Design review of the part built by this model. Coordinates are the model's own, in mm. Face numbers are marked on the shaded views. A direction names the side the tool comes from. Round coordinates to 2 decimals unless told otherwise and drop trailing zeros. Order: outer loops, then holes, each group sorted by start corner. A loop starts at its lowest first (then second) coordinate and runs counter-clockwise, first axis right, second up. Notation, with made-up numbers: (22, 7) - (55, 7) arc R13 cw to (55, 16) - close; hole circle Ø3 at (87.25, 39). An arc over 180 degrees is marked (long way). Write item = value, one per line.
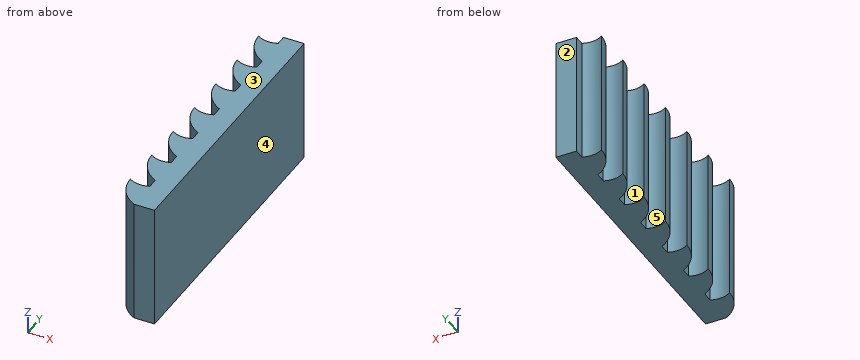
Autodesk Inventor part; units mm, degrees
ref_plane "YZ Plane" through (0, 0, 0) normal (1, 0, 0) x (0, 1, 0)
ref_plane "XZ Plane" through (0, 0, 0) normal (0, 1, 0) x (-1, 0, 0)
ref_plane "XY Plane" through (0, 0, 0) normal (0, 0, 1) x (1, 0, 0)
sketch "Sketch1" plane through (0, 0, 0) normal (0, 0, 1) x (1, 0, 0)
  line L0 (-3.81, 0) -> (0.635, 0)
  line L1 (0, -31.115) -> (0, 31.115)
  line L2 (0, -22.225) -> (0, 22.225)
  line L3 (0, -22.225) -> (-3.175, -22.225)
  line L4 (0, 22.225) -> (-3.175, 22.225)
  line L5 (-3.175, 22.225) -> (-3.175, -22.225) construction
  line L6 (-3.175, -22.225) -> (-3.175, 22.225)
  point P0 (0, 0)
  point P1 (0, 0)
  point P2 (-3.175, -18.1789)
  dimension "d0" = 44.45
  dimension "d3" = 3.175
extrude "Extrusion1" add sketch "Sketch1" along normal mid plane 19.05
sketch "Sketch2" plane through (0, 0, 0) normal (0, 0, 1) x (1, 0, 0)
  line L0 (-3.175, -22.225) -> (-3.175, 22.225)
  line L1 (0, -22.225) -> (-3.175, -22.225)
  line L2 (0, 22.225) -> (0, -22.225)
  line L3 (-3.175, 22.225) -> (0, 22.225)
  line L4 (-6.35, -22.225) -> (-6.35, 22.225) construction
  arc A0 (-6.35, -17.145) -> (-3.175, -22.225) centre (-0.6351, -17.1054) ccw
  arc A1 (-6.35, -17.145) -> (-3.175, -17.4625) centre (-4.4894, -14.5723) ccw
  line L5 (-6.35, -17.145) -> (0, -17.145) construction
  point P0 (0, 0)
  dimension "d10" = 3.175
  dimension "d11" = 5.08
  dimension "d12" = 5.715
  dimension "d14" = 3.175
  dimension "d15" = 0.3175
extrude "Extrusion2" add sketch "Sketch2" along normal mid plane 19.05 contours A0 A1 L0
pattern_linear "Rectangular Pattern1" count 7 spacing 6.35 along (0, 1, 0) of "Extrusion2"
properties part number "ratchet"
Item 1: Take a section at A-A, the plane x = -4. State the section outline as (y, z) points (3 decimals).
Data:
outline = (-21.725, -9.525) - (-17.709, -9.525) - (-17.709, 9.525) - (-21.725, 9.525) - close; (-15.375, -9.525) - (-11.359, -9.525) - (-11.359, 9.525) - (-15.375, 9.525) - close; (-9.025, -9.525) - (-5.009, -9.525) - (-5.009, 9.525) - (-9.025, 9.525) - close; (-2.675, -9.525) - (1.341, -9.525) - (1.341, 9.525) - (-2.675, 9.525) - close; (3.675, -9.525) - (7.691, -9.525) - (7.691, 9.525) - (3.675, 9.525) - close; (10.025, -9.525) - (14.041, -9.525) - (14.041, 9.525) - (10.025, 9.525) - close; (16.375, -9.525) - (20.391, -9.525) - (20.391, 9.525) - (16.375, 9.525) - close
Item 2: Take a section at D-D, the plane y = 17.5. State the section outline as (x, z) points (3 decimals), and give its area (3 significant figures).
Data:
outline = (-5.157, -9.525) - (0, -9.525) - (0, 9.525) - (-5.157, 9.525) - close
area = 98.2 mm2
Item 3: Insertion check: P1, Ø0.8, axis at y = -16.5, z = -2, coming from the -X side (3 decimals); P2, Ø3, axis at y = -13.5, z = 7, coming from the -X side. Each pin has a flat end and moves straight along its axis. Give the tip position at first contact, or say it passes through.
Data:
P1 = -3.175
P2 = -6.21
Item 4: For the marked faces 1 and 2, list the 3-axis set-ups (+Z, -Z, +X, -X, +Y, -Y) from which the entire face can be reached by the end or side of a thin tool; tool diameter is ignored.
Data:
face_1 = +Z, -Z
face_2 = +Z, -Z, +X, -X, +Y
Item 5: For line 1 along X through (y, z) = (-10.5, -6.25) (3 decimals); line 2 along X through (y, z) = (8, 6) (3 decimals); line 3 along X through (y, z) = (-12.5, -1.5), list the stretches that pass through material, from the lowest coordinate up. Write a range as [from, to].
Data:
line_1 = [-3.175, 0]
line_2 = [-6.343, -5.933], [-3.175, 0]
line_3 = [-6.08, 0]
Item 6: Take a section at C-C, the plane y = -5.5. State the section outline as (x, z) points (3 decimals).
Data:
outline = (-6.244, -9.525) - (0, -9.525) - (0, 9.525) - (-6.244, 9.525) - close
Item 7: The part is to be moulded in two halves that separate along X. For the marked faces 3, 4 and 5, say which applies: +X half, -X half, draft (parallel to the pull), parting line (faces both ways), or undercut.
Data:
face_3 = draft
face_4 = +X half
face_5 = undercut
